Geometry: final body of the model. Coordinates: model frame, mm. Face numbers are marked on the shaded views. A direction names the side the tool comes from. Round coordinates to 2 decimals unless told otherwise and drop trailing zeros. Loops run counter-clockwise (first coordinate to the right, second up) from the corner with the lowest first, then second, coordinate; pieces in that order, holes last. Notation, with made-up numbers: (-14.75, 20.5) - (28.25, 20.5) arc R15 ccw to (28.25, 28.5) - close; hole circle Ø7 at (30.25, 22). An arc over 180 degrees is marked (long way). Answer in a Markdown table with one row per item. Add a question column.
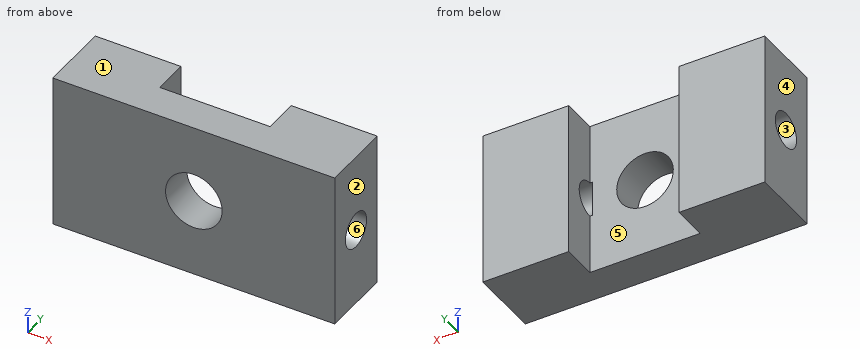
from build123d import *

# Parameters (mm, degrees)
SKETCH_1_W          = 79.688684702
SKETCH_1_H          = 43.973938876
SKETCH_1_R          = 8
EXTRUDE_1_DEPTH     = 20
SKETCH_2_R          = 5
CUT_EXTRUDE_2_DEPTH = 25
CUT_EXTRUDE_START   = -25
SKETCH_3_R          = 5
CUT_EXTRUDE_3_DEPTH = 25
SKETCH_4_W          = 31.2
SKETCH_4_H          = 50
CUT_EXTRUDE_4_DEPTH = 10


with BuildPart() as part:
    # Эскиз1 → Вытянуть1 (new body)
    with BuildSketch(Plane(origin=(0, 0, 0), x_dir=(1, 0, 0), z_dir=(0, 1, 0))):
        Rectangle(SKETCH_1_W, SKETCH_1_H)
        with Locations(Location((0, 0, 0), (0, 0, 270))):
            Circle(SKETCH_1_R, mode=Mode.SUBTRACT)
    extrude(amount=EXTRUDE_1_DEPTH)

    # Эскиз2 → Вытянуть2 (cut)
    with BuildSketch(Plane.ZY.offset(39.844342351)):
        with Locations((0, 10)):
            Circle(SKETCH_2_R)
    extrude(amount=-CUT_EXTRUDE_2_DEPTH, mode=Mode.SUBTRACT)

    # Эскиз3 → Вытянуть3 (cut)
    with BuildSketch(Plane(origin=(39.844342351, 0, 0), x_dir=(0, 0, -1), z_dir=(1, 0, 0)).offset(CUT_EXTRUDE_START)):
        with Locations(Location((0, 10, 0), (0, 0, 180))):
            Circle(SKETCH_3_R)
    extrude(amount=CUT_EXTRUDE_3_DEPTH, mode=Mode.SUBTRACT)

    # Эскиз4 → Вытянуть4 (cut)
    with BuildSketch(Plane(origin=(0, 20, 0), x_dir=(1, 0, 0), z_dir=(0, 1, 0))):
        Rectangle(SKETCH_4_W, SKETCH_4_H)
    extrude(amount=-CUT_EXTRUDE_4_DEPTH, mode=Mode.SUBTRACT)


solid = part.part
1) Section A-A, the plane z = 0. Return the cut outline in (x, y), and give its area (3 significant figures).
2) Contact query for flat-ended pins moving along their axis: pin 1 Ø2.5 at (y, z) = (8, -2) entering from -X; pin 2 Ø4 at (y, z) = (8.5, 1) entering from +X; pin 3 Ø13 at (x, z) = (0, 0) entering from +Y; pin 4 Ø15.5 at (x, z) = (-7, -4) entering from +Y. Output: stop coordinate, or through.
3) Pull-direction query (Z, two-part tool) for the marked faces 1, 2 and 3; classes: pulls with the +Z half, pulls with the -Z half, needs draft (parallel to the pull), parting line crosses it, or undercut.
4) Section B-B, the plane x = 0. Return the cut outline in (y, z), and give its area (3 significant figures).
5) Material intervals for line 1 along X through (y, z) = (11.5, 18.5); line 2 along Y through (x, z) = (-33.5, 0); line 3 along Z through (x, y) = (-34.5, 10), sorted ascending. Write a range as from..to.
6) Section D-D, the plane x = 20.5. Return the cut outline in (y, z), and give its area (3 significant figures).
7) Reachability of the marked faces 4, 5 and 6 from +Z, -Z, +X, -X, +Y, -Y: full face, straight path, thin tool, end or side. Return the list, or none.
8) Section C-C, the plane y = 16.5. Return the cut outline in (x, z).
Evaluation:
| question | item | result |
|---|---|---|
| 1 | outline | (-39.84, 0) - (-8, 0) - (-8, 10) - (-14.84, 10) - (-14.84, 5) - (-39.84, 5) - close; (-39.84, 15) - (-15.6, 15) - (-15.6, 20) - (-39.84, 20) - close; (8, 0) - (39.84, 0) - (39.84, 5) - (14.84, 5) - (14.84, 10) - (8, 10) - close; (15.6, 15) - (39.84, 15) - (39.84, 20) - (15.6, 20) - close |
| 1 | area | 629 mm² |
| 2 | pin 1 | stops at x = -14.84 |
| 2 | pin 2 | stops at x = 14.84 |
| 2 | pin 3 | passes through |
| 2 | pin 4 | stops at y = 10 |
| 3 | face 1 | pulls with the +Z half |
| 3 | face 2 | needs draft |
| 3 | face 3 | undercut |
| 4 | outline | (0, -21.99) - (10, -21.99) - (10, -8) - (0, -8) - close; (0, 8) - (10, 8) - (10, 21.99) - (0, 21.99) - close |
| 4 | area | 280 mm² |
| 5 | line 1 | x = -39.84..-15.6, 15.6..39.84 |
| 5 | line 2 | y = 0..5, 15..20 |
| 5 | line 3 | z = -21.99..-5, 5..21.99 |
| 6 | outline | (0, -21.99) - (20, -21.99) - (20, 21.99) - (0, 21.99) - close; hole circle Ø10 at (10, 0) |
| 6 | area | 801 mm² |
| 7 | face 4 | +Z, -Z, -X, +Y, -Y |
| 7 | face 5 | +Z, -Z, +Y |
| 7 | face 6 | +X |
| 8 | outline | (-39.84, -21.99) - (-15.6, -21.99) - (-15.6, 21.99) - (-39.84, 21.99) - close; (15.6, -21.99) - (39.84, -21.99) - (39.84, 21.99) - (15.6, 21.99) - close |
